Read the model definition and answer for the solid it produces. Units are mm, in the model's axes. A direction names the side the tool comes from. Coordinates: 2 decimals unless noted, no trailing zeros. Order: outer loops, then holes, each group sorted by start corner. A loop starts at its lowest first (then second) coordinate and runs counter-clockwise, first axis right, second up. Notation, with made-up numbers: (50.5, 40.25) -> (106.5, 40.25) arc R23 ccw to (106.5, 54.25) -> close; hole circle Ø1 at (-12.75, -33). An arc over 180 degrees is marked (long way). Return JSON: item names as keys, results as strings. Group by question number.
```python
from build123d import *

# Parameters (mm, degrees)
SKETCH_2_W       = 21.3
SKETCH_2_H       = 18.2
EXTRUDE_1_DEPTH  = 1.7
SKETCH_4_W       = 21.3
SKETCH_4_H       = 1.6
EXTRUDE_2_DEPTH  = 1.6
CHAMFER_1_SIZE   = 1.4
CHAMFER_1_SIZE_2 = 0.808290377
SKETCH_5_W       = 2.9
SKETCH_5_H       = 3.8
EXTRUDE_3_DEPTH  = 2
SKETCH_6_W       = 20
SKETCH_6_H       = 2.55
EXTRUDE_4_DEPTH  = 17.5


with BuildPart() as part:
    # 草图2 → 凸台-拉伸1 (new body)
    with BuildSketch(Plane(origin=(0, 0, 0), x_dir=(1, 0, 0), z_dir=(0, 1, 0))):
        Rectangle(SKETCH_2_W, SKETCH_2_H)
    extrude(amount=EXTRUDE_1_DEPTH)

    # 草图4 → 凸台-拉伸2 (add)
    with BuildSketch(Plane(origin=(0, 1.7, 0), x_dir=(1, 0, 0), z_dir=(0, 1, 0))):
        with Locations((0, 7.5)):
            Rectangle(SKETCH_4_W, SKETCH_4_H)
        with Locations((0, -7.5)):
            Rectangle(SKETCH_4_W, SKETCH_4_H)
    extrude(amount=EXTRUDE_2_DEPTH)

    # 倒角1
    # the kernel refuses this chamfer: 1.4, 0.808290377 mm, written as the material it takes off along each edge
    with BuildSketch(Plane(origin=(14.271920057, 3.3, 8.3), x_dir=(0, -0.9998132206222079, 0.019326765612701028), z_dir=(-1, 0, 0)), Plane(origin=(-14.271920057, 3.3, 6.7), x_dir=(0, -0.9998132206222079, -0.019326765612701028), z_dir=(1, 0, 0)), Plane(origin=(14.271920057, 3.3, -6.7), x_dir=(0, -0.9998132206222079, 0.019326765612701028), z_dir=(-1, 0, 0)), Plane(origin=(-14.271920057, 3.3, -8.3), x_dir=(0, -0.9998132206222079, -0.019326765612701028), z_dir=(1, 0, 0))) as chamfer_1_piece_1:
        Polygon((CHAMFER_1_SIZE * 0.999813220622, -CHAMFER_1_SIZE * 0.0193267656127), (-CHAMFER_1_SIZE_2 * 0.0193267656095, -CHAMFER_1_SIZE_2 * 0.999813220456), (0, 0), align=None)
    extrude(amount=28.543840113, mode=Mode.SUBTRACT)

    # 草图5 → 凸台-拉伸3 (add)
    with BuildSketch(Plane(origin=(0, 1.7, 0), x_dir=(1, 0, 0), z_dir=(0, 1, 0))):
        with Locations((8.2, 0)):
            Rectangle(SKETCH_5_W, SKETCH_5_H)
    extrude(amount=EXTRUDE_3_DEPTH)

    # 草图6 → 凸台-拉伸4 (add)
    with BuildSketch(Plane.XZ):
        with Locations((0, -7.65)):
            Rectangle(SKETCH_6_W, SKETCH_6_H)
        with Locations((0, 7.65)):
            Rectangle(SKETCH_6_W, SKETCH_6_H)
    extrude(amount=EXTRUDE_4_DEPTH)


solid = part.part
```
1. Which of the six approach directions +Z, -Z, +X, -X, +Y, -Y give full straight-line access (tool end or side, diameter ignored) to faces 5 (the face through (8, 3.7, 0)), 6 (the face through (-10, -9, -8)), 7 (the face through (8, 3, 1.9)), 8 (the face through (10, -9, -8)), 9 (the face through (0, -9, 8.925))?
2. Find section B-B on z = 0.75. Determine the outline of the cut face in (x, y), and give its area (3 significant figures).
3. Find section A-A on y = -4. Determine the outline of the cut face in (x, z) (3 decimals).
4. Straight lines are drawn through the part: L1, parallel to Z at x = 5, y = -11 (3 decimals); L2, parallel to X at y = -11.75, z = 6.5; L3, parallel to Y at x = 4.25, z = 0.25. For each, find the intervals that lie inside material, in ascending order.
5. Given pin 1 (1.5 mm diameter, centred on x = -3.5, y = -13.5, fed in from -Z) (3 decimals); pin 2 (3 mm diameter, centred on x = -5, y = -11, fed in from +Z) (3 decimals); pin 3 (5.5 mm diameter, centred on x = -1, z = -2, fed in from -Y), each flat-ended and moving along its own axis, determine where each tip first touches the part or whether it passes through.
6. Find section D-D on x = 4. Determine the outline of the cut face in (y, z) (3 decimals), and give its area (3 significant figures).
7. Find section C-C on x = 8.75. Determine the outline of the cut face in (y, z) (3 decimals).
8. For a pull along Z with two mould halves and no side action, classify faces 1 (the face through (9.65, 3, 0)), 2 (the face through (0, 1, 9.1)), 3 (the face through (0, -9, -6.375)), 4 (the face through (0, -17.5, -8)) as released by +Z, released by -Z, zero draft, split by the parting line, or undercut.
Result:
{
 "1": {"face 5": "+Z, -Z, +X, -X, +Y", "face 6": "+Z, -Z, -X, -Y", "face 7": "+X, -X, +Y", "face 8": "+Z, -Z, +X, -Y", "face 9": "+Z, +X, -X, -Y"},
 "2": {"outline": "(-10.65, 0) -> (10.65, 0) -> (10.65, 1.7) -> (9.65, 1.7) -> (9.65, 3.7) -> (6.75, 3.7) -> (6.75, 1.7) -> (-10.65, 1.7) -> close", "area": "42.0 mm^2"},
 "3": {"outline": "(-10, -8.925) -> (10, -8.925) -> (10, -6.375) -> (-10, -6.375) -> close; (-10, 6.375) -> (10, 6.375) -> (10, 8.925) -> (-10, 8.925) -> close"},
 "4": {"L1": "-8.925 to -6.375, 6.375 to 8.925", "L2": "-10 to 10", "L3": "0 to 1.7"},
 "5": {"pin 1": "z = -8.925", "pin 2": "z = 8.925", "pin 3": "y = 0"},
 "6": {"outline": "(-17.5, -8.925) -> (0, -8.925) -> (0, -9.1) -> (1.7, -9.1) -> (1.7, -8.3) -> (1.9, -8.3) -> (3.286, -7.5) -> (1.9, -6.7) -> (1.7, -6.7) -> (1.7, 6.7) -> (1.9, 6.7) -> (3.286, 7.5) -> (1.9, 8.3) -> (1.7, 8.3) -> (1.7, 9.1) -> (0, 9.1) -> (0, 8.925) -> (-17.5, 8.925) -> (-17.5, 6.375) -> (0, 6.375) -> (0, -6.375) -> (-17.5, -6.375) -> close", "area": "123 mm^2"},
 "7": {"outline": "(-17.5, -8.925) -> (0, -8.925) -> (0, -9.1) -> (1.7, -9.1) -> (1.7, -8.3) -> (1.9, -8.3) -> (3.286, -7.5) -> (1.9, -6.7) -> (1.7, -6.7) -> (1.7, -1.9) -> (3.7, -1.9) -> (3.7, 1.9) -> (1.7, 1.9) -> (1.7, 6.7) -> (1.9, 6.7) -> (3.286, 7.5) -> (1.9, 8.3) -> (1.7, 8.3) -> (1.7, 9.1) -> (0, 9.1) -> (0, 8.925) -> (-17.5, 8.925) -> (-17.5, 6.375) -> (0, 6.375) -> (0, -6.375) -> (-17.5, -6.375) -> close"},
 "8": {"face 1": "undercut", "face 2": "released by +Z", "face 3": "undercut", "face 4": "zero draft"}
}
